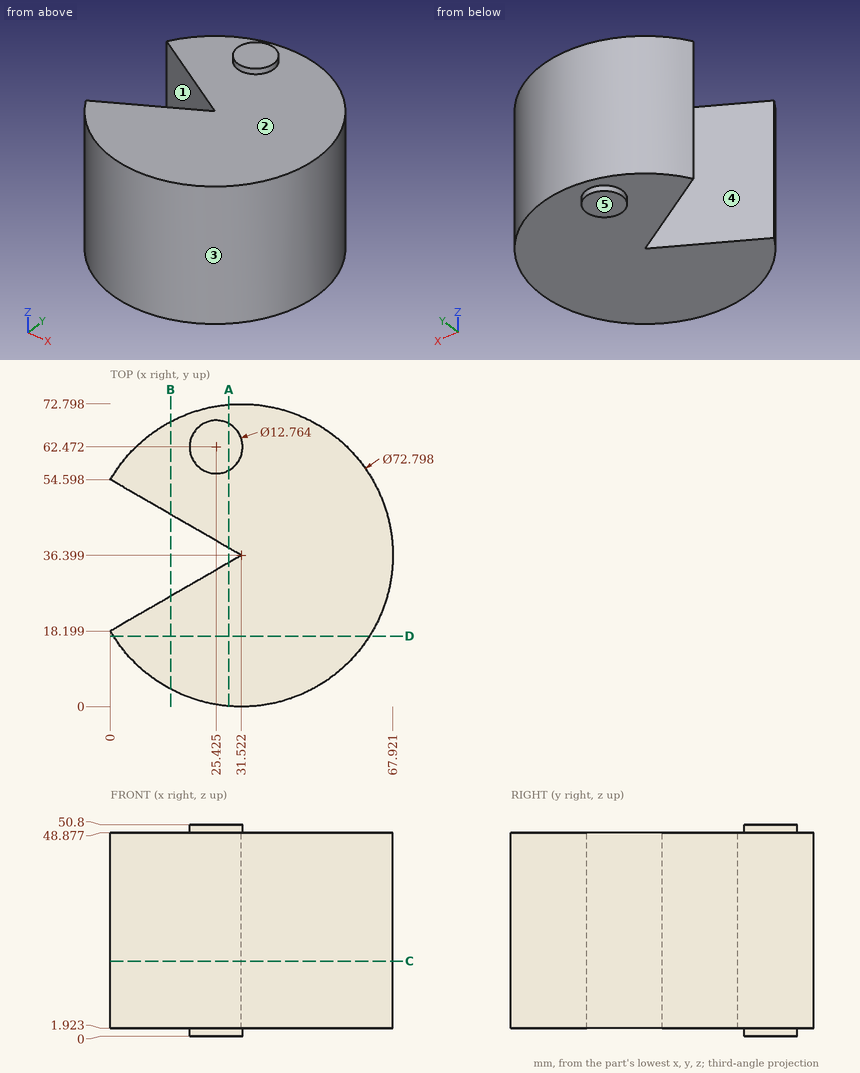
Could you check a few things on this drawing? It's one solid part, dimensions in mm from its lowest x, y, z. A direction names the side the tool comes from. Round coordinates to 2 decimals unless told otherwise and drop trailing zeros. Write each loop counter-clockwise with the first axis right and the second up, starting at its lowest first coordinate (ties: lowest second). Pieces come first, ordered by that corner, then holes. Notation, with made-up numbers: (-37, 34) -> (-23, 34) arc R22 cw to (-23, 50) -> close; hole circle Ø2 at (78.5, 3). An arc over 180 degrees is marked (long way). Use a Markdown table: item, result.
1. Please list where these lines run through material, in increasing order: probe 1 along Z at (x, y) = (32, 33.5); probe 2 along Y at (x, z) = (7, 43.5) (1 decimal); probe 3 along Y at (x, z) = (9, 3) (1 decimal).
Answer key:
| item | result |
|---|---|
| probe 1 | z = 1.92 to 48.88 |
| probe 2 | y = 9.5 to 22.2, 50.6 to 63.3 |
| probe 3 | y = 7.8 to 23.4, 49.4 to 65 |
2. If we section it at D-D (y = 17): List the corners of the cut face in (x, z) for me, then the cut area to 3 significant figures.
Answer key:
| item | result |
|---|---|
| outline | (0.72, 1.92) -> (62.32, 1.92) -> (62.32, 48.88) -> (0.72, 48.88) -> close |
| area | 2,890 mm^2 |
3. If we section it at C-C (z = 18): List the corners of the cut face in (x, y) for me, then the cut area to 3 significant figures.
Answer key:
| item | result |
|---|---|
| outline | (0, 18.2) arc R36.4 ccw (long way) to (0, 54.6) -> (31.52, 36.4) -> close |
| area | 3,470 mm^2 |
4. We'd pull the mould along Y, two halves only. Please class the marked faces 1, 2 and 3: +Y half, -Y half, draft (parallel to the pull), parting line (faces both ways), or undercut.
Answer key:
| item | result |
|---|---|
| face 1 | undercut |
| face 2 | draft |
| face 3 | parting line |
5. For pin 1 Ø2 at (x, z) = (60, 18) entering from +Y; pin 2 Ø8 at (y, z) = (65, 32) entering from -X (1 decimal); pin 3 Ø4 at (y, z) = (21, 29) entering from -X (1 decimal), each with a flat end and sliding along its axis, tell me the tip position at first contact or that it passes through.
Answer key:
| item | result |
|---|---|
| pin 1 | stops at y = 60.27 |
| pin 2 | stops at x = 4.7 |
| pin 3 | stops at x = 1.4 |
6. If we section it at A-A (x = 28.5): List the corners of the cut face in (y, z) for me (1 decimal), then the cut area to 3 significant figures.
Answer key:
| item | result |
|---|---|
| outline | (0.1, 1.9) -> (34.7, 1.9) -> (34.7, 48.9) -> (0.1, 48.9) -> close; (38.1, 1.9) -> (56.9, 1.9) -> (56.9, 0) -> (68.1, 0) -> (68.1, 1.9) -> (72.7, 1.9) -> (72.7, 48.9) -> (68.1, 48.9) -> (68.1, 50.8) -> (56.9, 50.8) -> (56.9, 48.9) -> (38.1, 48.9) -> close |
| area | 3,290 mm^2 |
7. If we section it at B-B (x = 14.5): List the corners of the cut face in (y, z) for me (1 decimal).
Answer key:
| item | result |
|---|---|
| outline | (4.2, 1.9) -> (26.6, 1.9) -> (26.6, 48.9) -> (4.2, 48.9) -> close; (46.2, 1.9) -> (68.6, 1.9) -> (68.6, 48.9) -> (46.2, 48.9) -> close |
8. Which directions (+Z, -Z, +X, -X, +Y, -Y) give clear straight access to the entire face, cutting with the end or side of a thin tool? Please do the marked faces 4 and 5.
Answer key:
| item | result |
|---|---|
| face 4 | +Z, -Z, -X |
| face 5 | -Z, +X, -X, +Y, -Y |
